Geometry: final body of the model. Coordinates: model frame, mm. A direction names the side the tool comes from. Coordinates: 2 decimals unless noted, no trailing zeros. Loops run counter-clockwise (first coordinate to the right, second up) from the corner with the lowest first, then second, coordinate; pieces in that order, holes last. Notation, with made-up numbers: (-37.5, 5) -> (-7.5, 5) arc R23 ccw to (-7.5, 27) -> close; hole circle Ø2 at (66.25, 51.5). An arc over 180 degrees is marked (long way). One line per item, written item: value. Start each with the question number.
Item 1: Set-up query: faces 4 (the cylindrical face through (55.48, 417.79, 4.93)), 5 (the flat face through (250.137, 515.522, 4.93)). Return all of +Z, -Z, +X, -X, +Y, -Y with unobstructed straight access to the full face (end or side cutting, diameter ignored); none if empty.
Item 2: Section query B-B on y = 390. Return loops of the section in (x, z), then the cut area to 3 significant figures.
Item 3: Mould query, pull axis Y, two halves, no side actions, for faces 1 (the cylindrical face through (174.1, 272.2, 4.9)), 2 (the flat face through (64.76, 369.91, 4.93)), 3 (the cylindrical face through (103.7, 507.274, 4.93)). Classes: +Y half, -Y half, draft (parallel to the pull), parting line (faces both ways), or undercut.
Item 4: Section query A-A on x = 186. Return loops of the section in (y, z), then the cut area to 3 significant figures.
Item 5: Contact query for flat-ended pins moving along their axis: pin 1 Ø4 at (y, z) = (377, 2.5) entering from +X; pin 2 Ø2 at (y, z) = (483, 7) entering from -X; pin 3 Ø2 at (y, z) = (347, 7) entering from +X. Output: stop coordinate, or through.
Item 6: Section query D-D on y = 506.5. Return loops of the section in (x, z), then the cut area to 3 significant figures.
Item 7: Section query C-C on z = 1.75. Give the number of separate pieces and of enclosed holes in the cut face, then the cut area to 3 significant figures.
Item 8: Ray query, probe 1 along Y at (x, z) = (187, 7); probe 2 along X at (y, z) = (463.5, 5.5); probe 3 along Y at (x, z) = (303, 3.75). Return the intervals inside material, ascending. Write a range as from..to.
from build123d import *

# Parameters (mm, degrees)
EXTRUDE_1_DEPTH          = 10
PATTERN_CIRCULAR_1_COUNT = 8


with BuildPart() as part:
    # Sketch 1 → Extrude 1 (new body)
    with BuildSketch(Plane.XY):
        with BuildLine():
            Line((142.543194713, 319.58457711), (129.866098291, 295.745717525))
            Line((129.866098291, 295.745717525), (132.514860467, 294.337151256))
            Line((132.514860467, 294.337151256), (128.28916166, 286.390864728))
            Line((128.28916166, 286.390864728), (125.640399483, 287.799430997))
            Line((125.640399483, 287.799430997), (124.701355304, 286.033589546))
            ThreePointArc((124.701355304, 286.033589546), (174.869094963, 272.123990236), (226.769655421, 276.199634915))
            Line((226.769655421, 276.199634915), (226.185021463, 278.112277886))
            Line((226.185021463, 278.112277886), (223.316057006, 277.23532695))
            Line((223.316057006, 277.23532695), (220.685204199, 285.842220321))
            Line((220.685204199, 285.842220321), (223.554168656, 286.719171257))
            Line((223.554168656, 286.719171257), (215.661610233, 312.539851371))
            ThreePointArc((215.661610233, 312.539851371), (178.350963885, 308.262904384), (142.543194713, 319.58457711))
        make_face()
    extrude_1 = extrude(amount=EXTRUDE_1_DEPTH)

    # Pattern Circular 1: Extrude 1 ×8 about axis
    pattern_circular_1_axis = Axis((187.606138684, 404.323949445, 0), (0, 0, 1))
    for i in range(1, PATTERN_CIRCULAR_1_COUNT):
        add(extrude_1.rotate(pattern_circular_1_axis, i * 360 / PATTERN_CIRCULAR_1_COUNT))


solid = part.part
Reply:
1. face 4: +Z, -Z, -X
1. face 5: +Z, -Z
2. outline: (55.25, 0) -> (92.38, 0) -> (92.38, 10) -> (55.25, 10) -> close; (283.03, 0) -> (319.64, 0) -> (319.64, 10) -> (283.03, 10) -> close
2. area: 737 mm²
3. face 1: -Y half
3. face 2: undercut
3. face 3: +Y half
4. outline: (271.47, 0) -> (307.85, 0) -> (307.85, 10) -> (271.47, 10) -> close; (500.77, 0) -> (537.22, 0) -> (537.22, 10) -> (500.77, 10) -> close
4. area: 728 mm²
5. pin 1: stops at x = 318.05
5. pin 2: stops at x = 79.25
5. pin 3: stops at x = 308.84
6. outline: (102.76, 0) -> (272.86, 0) -> (272.86, 10) -> (102.76, 10) -> close
6. area: 1,700 mm²
7. separate pieces: 1
7. enclosed holes: 9
7. area: 26,200 mm²
8. probe 1: y = 271.45..307.85, 500.79..537.21
8. probe 2: x = 67.6..69.94, 79.79..111.59, 263.84..306.95
8. probe 3: y = 336.71..340.23, 346.36..470.51
